Could you check a few things on this model? Use its own coordinates, in mm. Face numbers are marked on the shaded views. Coordinates: 2 decimals unless noted, no trailing zeros. Order: outer loops, then holes, each group sorted by start corner. A loop starts at its lowest first (then second) coordinate and runs counter-clockwise, first axis right, second up. Notation, with made-up numbers: (36.25, 57.5) - (72.25, 57.5) arc R16 cw to (72.25, 78.5) - close; hole circle Ø7 at (64, -6.5). An arc over 180 degrees is marked (long way). One line per item, written item: value.
from build123d import *

# Parameters (mm, degrees)
CYLINDER003_R     = 11
CYLINDER003_DEPTH = 80
CYLINDER002_R     = 13
CYLINDER002_DEPTH = 67
CHAMFER001_SIZE   = 1
CYLINDER001_R     = 15
CYLINDER001_DEPTH = 11
CYLINDER_R        = 33
CYLINDER_DEPTH    = 2
CHAMFER002_SIZE   = 1
BOX_W             = 64
BOX_H             = 3
BOX_DEPTH         = 7
BOX001_W          = 64
BOX001_H          = 6
BOX001_DEPTH      = 3
CHAMFER_SIZE      = 1


with BuildPart() as cylinder003:
    # Cylinder003 → Cylinder003 (new body)
    with BuildSketch(Plane.XY.offset(-1)):
        Circle(CYLINDER003_R)
    extrude(amount=CYLINDER003_DEPTH)


with BuildPart() as chamfer001:
    # Cylinder002 → Cylinder002 (new body)
    with BuildSketch(Plane.XY.offset(10)):
        Circle(CYLINDER002_R)
    extrude(amount=CYLINDER002_DEPTH)

    # Chamfer001
    chamfer001_edges = [chamfer001.edges().sort_by_distance(p)[0] for p in [
        (-13, 0, 77),
    ]]
    chamfer(chamfer001_edges, length=CHAMFER001_SIZE)


with BuildPart() as chamfer001_1:
    # Chamfer001 placement: moved
    add(chamfer001.part.moved(Location((0, 0, -5))))


with BuildPart() as cylinder001:
    # Cylinder001 → Cylinder001 (new body)
    with BuildSketch(Plane.XY.offset(1)):
        Circle(CYLINDER001_R)
    extrude(amount=CYLINDER001_DEPTH)


with BuildPart() as chamfer002:
    # Cylinder → Cylinder (new body)
    with BuildSketch(Plane.XY):
        Circle(CYLINDER_R)
    extrude(amount=CYLINDER_DEPTH)

    # Fusion: union Cylinder001
    add(cylinder001.part)

    # Fusion001: union Chamfer001
    add(chamfer001_1.part)

    # Cut: cut Cylinder003
    add(cylinder003.part, mode=Mode.SUBTRACT)

    # Chamfer002
    chamfer002_edges = [chamfer002.edges().sort_by_distance(p)[0] for p in [
        (-33, 0, 2),
    ]]
    chamfer(chamfer002_edges, length=CHAMFER002_SIZE)


with BuildPart() as cube:
    # Box → Box (new body)
    with BuildSketch(Plane(origin=(-32, 0, -6), x_dir=(1, 0, 0), z_dir=(0, 0, 1))):
        with Locations((32, 1.5)):
            Rectangle(BOX_W, BOX_H)
    extrude(amount=BOX_DEPTH)


with BuildPart() as fusion003:
    # Box001 → Box001 (new body)
    with BuildSketch(Plane(origin=(-32, -4, -6), x_dir=(1, 0, 0), z_dir=(0, 0, 1))):
        with Locations((32, 3)):
            Rectangle(BOX001_W, BOX001_H)
    extrude(amount=BOX001_DEPTH)

    # Chamfer
    chamfer_edges = [fusion003.edges().sort_by_distance(p)[0] for p in [
        (0, -4, -3),
    ]]
    chamfer(chamfer_edges, length=CHAMFER_SIZE)

    # Fusion002: union Cube
    add(cube.part)


with BuildPart() as fusion003_1:
    # Fusion002 placement: moved
    add(fusion003.part.moved(Location((0, -6, 0))))

    # Fusion003: union Chamfer002
    add(chamfer002.part)


solid = fusion003_1.part
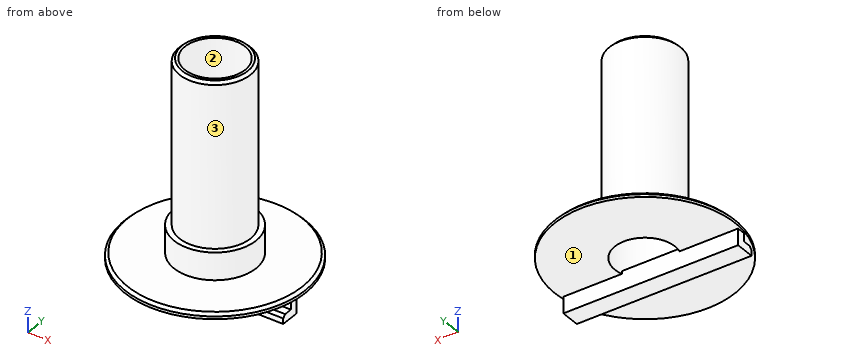
Item 1: If I drill on probe 1 along Y at (x, z) = (0, 38); probe 2 along Z at (x, y) = (-17, -5.5), over which ranges is the centre line in solid material (lowest first)?
Conclusion:
probe 1: -13 to -11, 11 to 13
probe 2: -6 to 2
Item 2: I want a section at D-D on z = 29. Please give me the cut outline in (x, y), then the cut area to 3 significant figures.
Conclusion:
outline: circle Ø26 at (0, 0); hole circle Ø22 at (0, 0)
area: 151 mm²
Item 3: I want a section at B-B on y = 0. Please give me the cut outline in (x, z).
Conclusion:
outline: (-33, 0) - (-11, 0) - (-11, 72) - (-12, 72) - (-13, 71) - (-13, 12) - (-15, 12) - (-15, 2) - (-32, 2) - (-33, 1) - close; (11, 0) - (33, 0) - (33, 1) - (32, 2) - (15, 2) - (15, 12) - (13, 12) - (13, 71) - (12, 72) - (11, 72) - close
Item 4: I'm going to push flat-ended pins straight in: pin 1 Ø6 at (x, y) = (-8, 24) entering from +Z; pin 2 Ø0.9 at (x, y) = (-5.5, -5) entering from +Z; pin 3 Ø3.5 at (x, z) = (-10.5, -2.5) entering from +Y. Where does each tip first touch, or does it pass through?
Conclusion:
pin 1: z = 2
pin 2: z = 1
pin 3: y = -3
Item 5: I want a section at C-C on z = 11. Please give me the cut outline in (x, y).
Conclusion:
outline: circle Ø30 at (0, 0); hole circle Ø22 at (0, 0)
Item 6: I want a section at A-A on x = 0. Please give me the cut outline in (y, z).
Conclusion:
outline: (-33, 0) - (-11, 0) - (-11, 72) - (-12, 72) - (-13, 71) - (-13, 12) - (-15, 12) - (-15, 2) - (-32, 2) - (-33, 1) - close; (-10, -6) - (-3, -6) - (-3, 1) - (-6, 1) - (-6, -3) - (-9, -3) - (-10, -4) - close; (11, 0) - (33, 0) - (33, 1) - (32, 2) - (15, 2) - (15, 12) - (13, 12) - (13, 71) - (12, 72) - (11, 72) - close
Item 7: Thinking about a two-plate mould opening in Y: for the marked faces 1, 2 and 3, which applies, pulls with the +Y half, pulls with the -Y half, needs draft (parallel to the pull), parting line crosses it, or undercut?
Conclusion:
face 1: needs draft
face 2: undercut
face 3: parting line crosses it
